Geometry check sheet. Reference: the model listing, model coordinates, mm. A direction names the side the tool comes from. Round coordinates to 2 decimals unless told otherwise and drop trailing zeros. Order: outer loops, then holes, each group sorted by start corner. A loop starts at its lowest first (then second) coordinate and runs counter-clockwise, first axis right, second up. Notation, with made-up numbers: (3.25, 84) -> (16.25, 84) arc R20 cw to (16.25, 94) -> close; hole circle Ø10 at (78, 39). An arc over 180 degrees is marked (long way). Use a Markdown table: item, result. Add a question column.
Item 1: Mould release check, pull along Y, two halves, no side actions. Record for faces 6 (the cylindrical face through (9.86, -4.57, 19.35)), 7 (the cylindrical face through (10.14, 3.449, 21.728)), 8 (the cylindrical face through (9.86, -15.037, -12.911)), 9 (the cylindrical face through (9.86, 7.678, 18.341)): pulls with the +Y half, pulls with the -Y half, needs draft (parallel to the pull), parting line crosses it, or undercut.
Item 2: Set-up check for faces 1 (the flat face through (0, 5, 0)), 2 (the cylindrical face through (9.86, 19.284, -4.576)), 3 (the cylindrical face through (9.86, 12.97, 15.07)), 4 (the cylindrical face through (10.14, -3.43, 21.73)), 5 (the cylindrical face through (9.86, -12.97, -15.07)): record each of +Z, -Z, +X, -X, +Y, -Y from which the full face is reachable in a straight line by a thin tool's end or side.
Item 3: Gauge pin test, flat ends, axial feed: pin 1 Ø5 at (x, y) = (4, 9) entering from -Z; pin 2 Ø1.5 at (x, y) = (14, 11) entering from -Z; pin 3 Ø1.9 at (x, z) = (11.5, -1) entering from -Y. Record the tip position at first contact, or that the pin passes through.
Item 4: Material ranges on probe 1 along Z at (x, y) = (5.25, 19); probe 2 along Y at (x, z) = (19.25, 15); probe 3 along Z at (x, y) = (7.5, -14), recorded low to high. Write a range as [from, to].
Item 5: Sectioned sample at A-A, the plane y = 8. Record the cut outline in (x, z).
from build123d import *

# Parameters (mm, degrees)
BASPROSKE_W        = 20
BASPROSKE_H        = 22
TOOTHCUT_DEPTH     = 37.986484018
TEETHCUTS_COUNT    = 20
TEETHCUTS_ANGLE    = 342
CUT_EXTRUDE1_DEPTH = 37.75639264


with BuildPart() as part:
    # BasProSke → Base-Revolve (revolve)
    with BuildSketch(Plane(origin=(0, 0, 0), x_dir=(1, 0, 0), z_dir=(0, 1, 0)), mode=Mode.PRIVATE) as base_revolve_sk:
        with Locations((10, 11)):
            Rectangle(BASPROSKE_W, BASPROSKE_H)
    revolve(base_revolve_sk.sketch.rotate(Axis((-10, 0, 0), (1, 0, 0)), 180), axis=Axis((-10, 0, 0), (1, 0, 0)))

    # TooCutSke → ToothCut (cut, through all)
    with BuildSketch(Plane(origin=(0, 0, 0), x_dir=(0, 0, -1), z_dir=(1, 0, 0))):
        with BuildLine():
            ThreePointArc((0.986171591, 17.471189616), (0, 17.499), (-0.986171591, 17.471189616))
            ThreePointArc((-0.986171591, 17.471189616), (-1.626916196, 19.798789858), (-2.932850173, 21.829260982))
            ThreePointArc((-2.932850173, 21.829260982), (0, 22.0254), (2.932850173, 21.829260982))
            ThreePointArc((2.932850173, 21.829260982), (1.626916196, 19.798789858), (0.986171591, 17.471189616))
        make_face()
    toothcut = extrude(amount=TOOTHCUT_DEPTH, mode=Mode.SUBTRACT)

    # TeethCuts: ToothCut ×20 about axis
    teethcuts_axis = Axis((-10, 0, 0), (1, 0, 0))
    for i in range(1, TEETHCUTS_COUNT):
        add(toothcut.rotate(teethcuts_axis, i * TEETHCUTS_ANGLE / (TEETHCUTS_COUNT - 1)), mode=Mode.SUBTRACT)

    # Sketch1 → Cut-Extrude1 (cut, through all)
    with BuildSketch(Plane(origin=(20, 0, 0), x_dir=(0, 0, -1), z_dir=(1, 0, 0))):
        with BuildLine():
            Line((1.907223112, 2.05), (-1.907223112, 2.05))
            ThreePointArc((-1.907223112, 2.05), (-2.8, 0), (-1.907223112, -2.05))
            Line((-1.907223112, -2.05), (1.907223112, -2.05))
            ThreePointArc((1.907223112, -2.05), (2.567121415, -1.11798374), (2.8, 0))
            ThreePointArc((2.8, 0), (2.567121415, 1.11798374), (1.907223112, 2.05))
        make_face()
    extrude(amount=-CUT_EXTRUDE1_DEPTH, mode=Mode.SUBTRACT)


solid = part.part
Found:
| question | item | result |
|---|---|---|
| 1 | face 6 | undercut |
| 1 | face 7 | pulls with the +Y half |
| 1 | face 8 | pulls with the -Y half |
| 1 | face 9 | undercut |
| 2 | face 1 | +Z, -Z, -X, +Y, -Y |
| 2 | face 2 | +X, -X |
| 2 | face 3 | +Z, +X, -X |
| 2 | face 4 | +Z, +X, -X, -Y |
| 2 | face 5 | -Z, +X, -X |
| 3 | pin 1 | stops at z = -19.84 |
| 3 | pin 2 | stops at z = -19.47 |
| 3 | pin 3 | stops at y = -20.44 |
| 4 | probe 1 | z = [-10.49, -8.35], [-4.6, -1.32], [1.32, 4.6], [8.35, 10.49] |
| 4 | probe 2 | y = [-15.89, -12.85], [-9.62, 9.62], [12.85, 15.89] |
| 4 | probe 3 | z = [-15.57, -11.51], [-10.5, 10.5], [11.51, 15.57] |
| 5 | outline | (0, -18.68) -> (20, -18.68) -> (20, 18.68) -> (0, 18.68) -> close |
